Autodesk Inventor part; units mm, degrees
ref_plane "Work Plane2" through (0, 0, 1.5) normal (0, 0, 1) x (1, 0, 0)
ref_plane "Work Plane8" through (0, 0, 0) normal (0.9238795, 0.3826834, 0) x (0, 0, 1)
ref_plane "Work Plane9" through (0, 0, 0) normal (1, 0, 0) x (0, 1, 0)
sketch "Sketch1" plane through (0, 0, 0) normal (0, 0, 1) x (1, 0, 0)
  circle A0 centre (0, 0) radius 10
  dimension "d0" = 20
extrude "Extrusion1" add sketch "Sketch1" along normal blind 3
ref_plane "Work Plane2" through (0, 0, 1.5) normal (0, 0, 1) x (1, 0, 0)
sketch "Sketch2" plane through (0, 0, 0) normal (0, 0, -1) x (-1, 0, 0)
  circle A0 centre (0, 0) radius 10
  circle A1 centre (0, 0) radius 8
  dimension "d3" = 16
surface extrude "Pitch Diameter" sketch "Sketch2" against normal through all shown no curves A1
ref_plane "Work Plane8" through (0, 0, 0) normal (0.9238795, 0.3826834, 0) x (0, 0, 1)
ref_plane "Work Plane9" through (0, 0, 0) normal (1, 0, 0) x (0, 1, 0)
spur gear teeth "Spur Gear" teeth 8 pitch diameter 16 tip diameter 20 root diameter 11 face width 3 start plane through (0, 0, 0) normal (0, 0, -1) x (-1, 0, 0)
sketch "Sketch3" plane through (0, 0, 3) normal (0, 0, 1) x (1, 0, 0)
  circle A0 centre (0, 0) radius 3
  dimension "d49" = 6
extrude "Extrusion2" cut sketch "Sketch3" against normal blind 1
sketch "Sketch4" plane through (0, 0, 2) normal (0, 0, 1) x (1, 0, 0)
  circle A0 centre (0, 0) radius 1.5
  dimension "d52" = 3
extrude "Extrusion3" cut sketch "Sketch4" against normal blind 2
equation "\"d0\" = da_da"
equation "\"d1\" = da_b"
equation "\"d3\" = da_d"
equation "\"d16\" = da_aw"
equation "\"d43\" = da_aw"
equation "\"d46\" = da_aw"
properties part number "engrenagem8_3_furo_3DPrint"
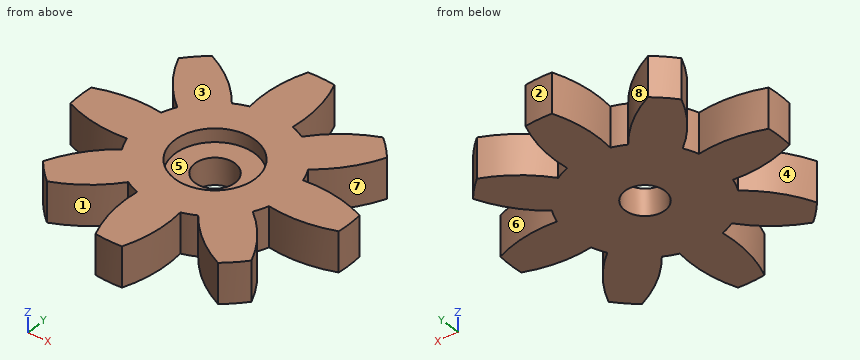
Here's how the part is built. I have some questions about the finished solid (model axes, mm). Face numbers are marked on the shaded views. A direction names the side the tool comes from. Round coordinates to 2 decimals unless told otherwise and drop trailing zeros. Order: outer loops, then holes, each group sorted by start corner. A loop starts at its lowest first (then second) coordinate and runs counter-clockwise, first axis right, second up. Notation, with made-up numbers: M 77,46 L 124,46 A28 ccw 124,65 Z; hole C 23.5,31.25 d3. An arc over 180 degrees is marked long. Answer in a Markdown table with one row per item.
Item 1: Imagine slicing it at B-B, the plane x = 0. Write out the boundary of the cut face in (y, z), and give its area (3 significant figures).
A:
| item | result |
|---|---|
| outline | M -10,0 L -1.5,0 L -1.5,2 L -3,2 L -3,3 L -10,3 Z; M 1.5,0 L 10,0 L 10,3 L 3,3 L 3,2 L 1.5,2 Z |
| area | 48.0 mm2 |
Item 2: For the marked faces 4, 5, 6, 7 and 8, which set-ups out of +Z, -Z, +X, -X, +Y, -Y let a thin tool reach every point of the face, with its end or its side?
A:
| item | result |
|---|---|
| face 4 | +Z, -Z, -X |
| face 5 | +Z |
| face 6 | +Z, -Z |
| face 7 | +Z, -Z, +X |
| face 8 | +Z, -Z, +Y |
Item 3: Thinking about a two-plate mould opening in X: for the marked faces 1, 2 and 3, which applies, +X half, -X half, draft (parallel to the pull), parting line (faces both ways), or undercut?
A:
| item | result |
|---|---|
| face 1 | undercut |
| face 2 | parting line |
| face 3 | draft |
Item 4: If I drill on L1, parallel to Y at x = 0, z = 0.8; L2, parallel to Y at x = 0, z = 2.3; L3, parallel to X at y = 5.5, z = 1.3, over which ranges is the centre line in solid material (lowest first)? Write a range as from..to.
A:
| item | result |
|---|---|
| L1 | y = -10..-1.5, 1.5..10 |
| L2 | y = -10..-3, 3..10 |
| L3 | x = -7.32..-3.15, -1.62..1.62, 3.15..7.32 |
Item 5: Imagine slicing it at D-D, the plane x = -7. Write out the boundary of the cut face in (y, z), and give its area (3 significant figures).
A:
| item | result |
|---|---|
| outline | M -7.14,0 L -4.95,0 L -4.95,3 L -7.14,3 Z; M -1.65,0 L 1.65,0 L 1.65,3 L -1.65,3 Z; M 4.95,0 L 7.14,0 L 7.14,3 L 4.95,3 Z |
| area | 23.0 mm2 |
Item 6: Imagine slicing it at C-C, the plane y = 0.5. Write out the boundary of the cut face in (x, z), and give its area (3 significant figures).
A:
| item | result |
|---|---|
| outline | M -9.99,0 L -1.41,0 L -1.41,2 L -2.96,2 L -2.96,3 L -9.99,3 Z; M 1.41,0 L 9.99,0 L 9.99,3 L 2.96,3 L 2.96,2 L 1.41,2 Z |
| area | 48.4 mm2 |
Item 7: I'm going to push flat-ended pins straight in: pin 1 (3 mm diameter, centred on x = 0.5, y = -1, fed in from +Z); pin 2 (2.5 mm diameter, centred on x = 0, y = 0, fed in from +Z); pin 3 (1.5 mm diameter, centred on y = 1.5, z = 2, fed in from -X). Where does each tip first touch, or does it pass through?
A:
| item | result |
|---|---|
| pin 1 | stops at z = 2 |
| pin 2 | passes through |
| pin 3 | stops at x = -9.97 |
